Design review of the part built by this model. Coordinates are the model's own, in mm. A direction names the side the tool comes from. Give positions to 0.01 mm unless a question says otherwise; leave off trailing zeros. Write each loop counter-clockwise with the first axis right and the second up, starting at its lowest first coordinate (ties: lowest second). Pieces come first, ordered by that corner, then holes. Notation, with made-up numbers: M -20.5,88 L -0.5,88 A14 ccw -0.5,112 Z; hole C 21.5,76 d5. An arc over 180 degrees is marked long. Answer in a Markdown table with one row per item.
```python
from build123d import *

# Parameters (mm, degrees)
SKETCH1_R           = 19.5
SKETCH1_R_2         = 10.5
BOSS_EXTRUDE1_DEPTH = 5
SKETCH3_R           = 4
BOSS_EXTRUDE2_DEPTH = 35
SKETCH4_R           = 1.25
CUT_EXTRUDE1_DEPTH  = 7


with BuildPart() as part:
    # Sketch1 → Boss-Extrude1 (new body)
    with BuildSketch(Plane.XY):
        Circle(SKETCH1_R)
        Circle(SKETCH1_R_2, mode=Mode.SUBTRACT)
    extrude(amount=BOSS_EXTRUDE1_DEPTH)

    # Sketch3 → Boss-Extrude2 (add)
    with BuildSketch(Plane.XY.offset(5)):
        with Locations((-15, 0)):
            Circle(SKETCH3_R)
        with Locations(Location((15, 0, 0), (0, 0, 180))):
            Circle(SKETCH3_R)
    extrude(amount=BOSS_EXTRUDE2_DEPTH)

    # Sketch4 → Cut-Extrude1 (cut)
    with BuildSketch(Plane.XY.offset(40)):
        with Locations((15, 0)):
            Circle(SKETCH4_R)
        with Locations((-15, 0)):
            Circle(SKETCH4_R)
    extrude(amount=-CUT_EXTRUDE1_DEPTH, mode=Mode.SUBTRACT)


solid = part.part
```
1) For faces 5 (the face through (10, 3.2, 2.5)), 6 (the face through (-16.25, 0.05, 36.55)), list the 3-axis set-ups (+Z, -Z, +X, -X, +Y, -Y) from which the entire face can be reached by the end or side of a thin tool; tool diameter is ignored.
Geometry says:
| item | result |
|---|---|
| face 5 | +Z, -Z |
| face 6 | +Z |
2) Add section A-A (x = 0). Write out the cut boundary in (y, z).
Geometry says:
| item | result |
|---|---|
| outline | M -19.5,0 L -10.5,0 L -10.5,5 L -19.5,5 Z; M 10.5,0 L 19.5,0 L 19.5,5 L 10.5,5 Z |
3) Add section B-B (y = 0). Write out the cut boundary in (x, z), and give its area (3 significant figures).
Geometry says:
| item | result |
|---|---|
| outline | M -19.5,0 L -10.5,0 L -10.5,5 L -11,5 L -11,40 L -13.75,40 L -13.75,33 L -16.25,33 L -16.25,40 L -19,40 L -19,5 L -19.5,5 Z; M 10.5,0 L 19.5,0 L 19.5,5 L 19,5 L 19,40 L 16.25,40 L 16.25,33 L 13.75,33 L 13.75,40 L 11,40 L 11,5 L 10.5,5 Z |
| area | 615 mm^2 |
4) Add section C-C (z = 12.5). Write out the cut boundary in (x, y), and give its area (3 significant figures).
Geometry says:
| item | result |
|---|---|
| outline | C -15,0 d8; C 15,0 d8 |
| area | 101 mm^2 |
5) Insertion check: P1, Ø12, axis at x = -7.5, z = 31.5, coming from the +Y side; P2, Ø0.8, axis at x = -15, y = -0.5, coming from the +Z side; P3, Ø3, axis at x = 4, y = 12, coming from the +Z side. Each pin has a flat end and moves straight along its axis. Give the tip position at first contact, or say it passes through.
Geometry says:
| item | result |
|---|---|
| P1 | y = 3.71 |
| P2 | z = 33 |
| P3 | z = 5 |
6) Add section D-D (y = -8.5). Write out the cut boundary in (x, z), and give its area (3 significant figures).
Geometry says:
| item | result |
|---|---|
| outline | M -17.55,0 L -6.16,0 L -6.16,5 L -17.55,5 Z; M 6.16,0 L 17.55,0 L 17.55,5 L 6.16,5 Z |
| area | 114 mm^2 |
7) The part is to be moulded in two halves that separate along X. For faces 1 (the face through (-2.539, 19.334, 2.465)), 2 (the face through (15, 0, 33)), 3 (the face through (8, -8, 0)), 4 (the face through (-15, 0, 33)), say which applies: released by +X, released by -X, zero draft, split by the parting line, or undercut.
Geometry says:
| item | result |
|---|---|
| face 1 | split by the parting line |
| face 2 | undercut |
| face 3 | zero draft |
| face 4 | undercut |
8) To check wall thickness, follow probe 1 along Y at (x, z) = (0, 3); probe 2 along Y at (x, z) = (-15, 38); probe 3 along Z at (x, y) = (-1, 16.5). State the ranges of each line that lie inside material, in increasing order. Write a range as [from, to].
Geometry says:
| item | result |
|---|---|
| probe 1 | [-19.5, -10.5], [10.5, 19.5] |
| probe 2 | [-4, -1.25], [1.25, 4] |
| probe 3 | [0, 5] |
